Study the drawing (mm; zero at the part's minimum x, y, z) and answer. A direction names the side the tool comes from. Give positions to 0.01 mm unless a question says otherwise; leave off trailing zeros. Write each loop counter-clockwise with the first axis right and the second up, starting at its lowest first coordinate (ties: lowest second). Pieces come first, ordered by that corner, then holes. Notation, with made-up numbers: (-21, 3) -> (-8, 3) arc R14 cw to (-8, 8) -> close; hole circle Ø7 at (-38, 43.5). An arc over 180 degrees is marked (long way). Put each result on its own line as item: value. Start each with the question number.
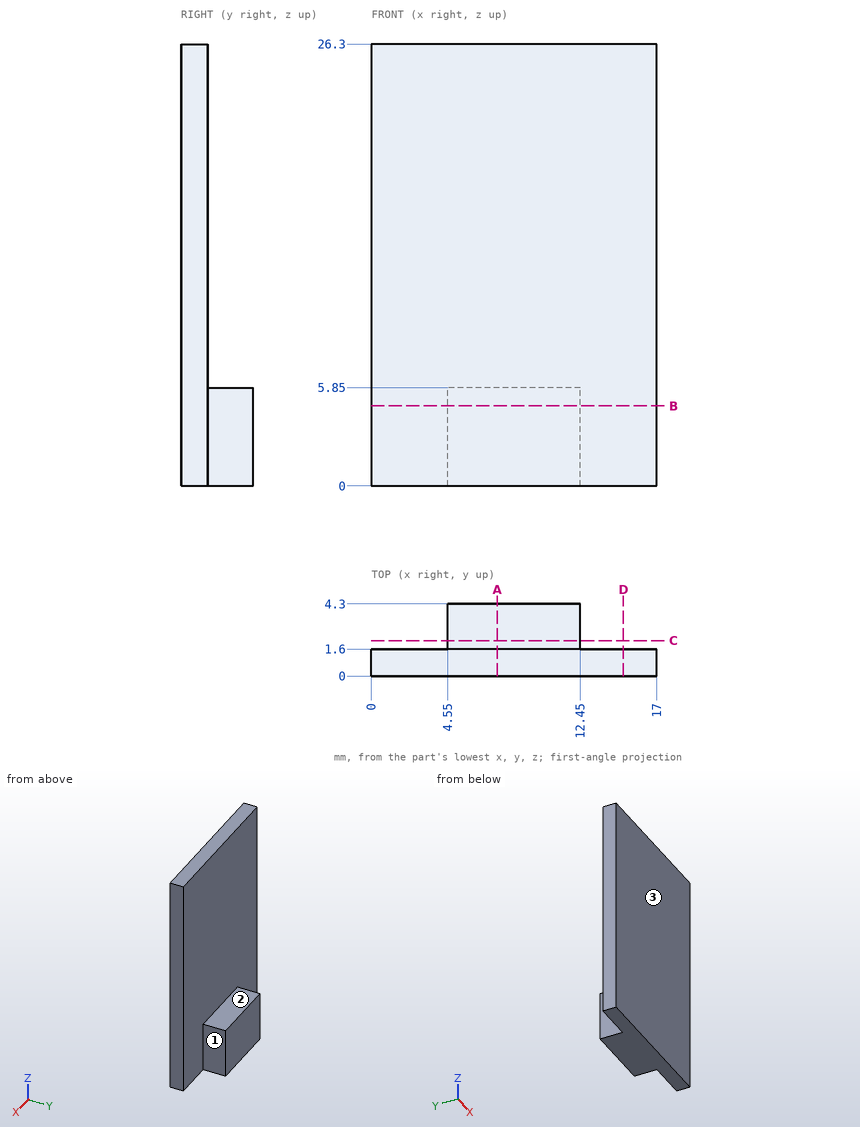
1) For the marked faces 1, 2 and 3, determine the directions among +Z, -Z, +X, -X, +Y, -Y from which every point of the face is accessible in a straight line to the end or side of a thin tool.
2) Each of these flat-tipped pins is pushed along its axis until it touches: pin 1 Ø0.8 at (x, y) = (8.5, 2.5) entering from +Z; pin 2 Ø5 at (x, z) = (2, 17) entering from +Y. Where does it stop, or does it pass through?
3) A cutting plane is placed at C-C on y = 2.1. Give the vertices of the cut face in (x, z), and give its area (3 significant figures).
4) Straight lines are drawn through the part: line 1 (Y direction, x = 8.75, z = 11); line 2 (Z direction, x = 9.5, y = 1.95); line 3 (X direction, y = 3.2, z = 4.75). For each, find the intervals that lie inside material, in ascending order. Write a range as [from, to].
5) A cutting plane is placed at A-A on x = 7.5. Give the vertices of the cut face in (y, z).
6) A cutting plane is placed at D-D on x = 15. Give the vertices of the cut face in (y, z).
7) A cutting plane is placed at B-B on z = 4.75. Give the vertices of the cut face in (x, y), and give its area (3 significant figures).
Results found:
1. face 1: +Z, -Z, +X, +Y
1. face 2: +Z, +X, -X, +Y
1. face 3: +Z, -Z, +X, -X, -Y
2. pin 1: stops at z = 5.85
2. pin 2: stops at y = 1.6
3. outline: (4.55, 0) -> (12.45, 0) -> (12.45, 5.85) -> (4.55, 5.85) -> close
3. area: 46.2 mm²
4. line 1: y = [0, 1.6]
4. line 2: z = [0, 5.85]
4. line 3: x = [4.55, 12.45]
5. outline: (0, 0) -> (4.3, 0) -> (4.3, 5.85) -> (1.6, 5.85) -> (1.6, 26.3) -> (0, 26.3) -> close
6. outline: (0, 0) -> (1.6, 0) -> (1.6, 26.3) -> (0, 26.3) -> close
7. outline: (0, 0) -> (17, 0) -> (17, 1.6) -> (12.45, 1.6) -> (12.45, 4.3) -> (4.55, 4.3) -> (4.55, 1.6) -> (0, 1.6) -> close
7. area: 48.5 mm²
